Work out the finished part from the listing and answer in its coordinate system (mm). Face numbers are marked on the shaded views. A direction names the side the tool comes from. Coordinates: 2 decimals unless noted, no trailing zeros. Write each loop counter-clockwise with the first axis right and the second up, starting at its lowest first coordinate (ties: lowest second). Pieces come first, ordered by that corner, then holes. Notation, with made-up numbers: (24, 53) - (68, 53) arc R25 ccw to (68, 73) - close; hole circle Ø1 at (37.25, 29). An arc over 180 degrees is marked (long way). One line per item, written item: value.
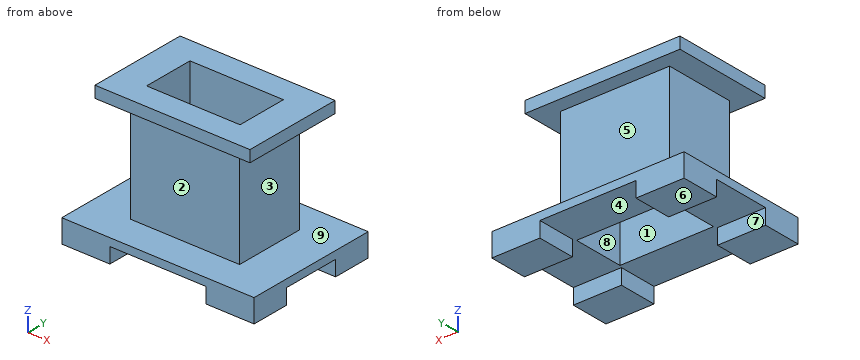
```python
from build123d import *

# Parameters (mm, degrees)
F0_W      = 127
F0_H      = 88.9
F1_DEPTH  = 15.24
F2_W      = 63.5
F2_H      = 10.16
F3_DEPTH  = 88.9
F4_W      = 38.1
F4_H      = 10.16
F5_DEPTH  = 127
F6_W      = 71.8820020556
F6_H      = 46.4872904122
F7_DEPTH  = 76.2
F8_W      = 61.7219954729
F8_H      = 33.7767079473
F9_DEPTH  = 101.6
F10_W     = 102.3619994521
F10_H     = 66.2887096405
F10_W_2   = 71.8820020556
F10_H_2   = 46.4872904122
F11_DEPTH = 7.62


with BuildPart() as f1:
    # F0 (on Top) → F1 (new body)
    with BuildSketch(Plane.XY):
        Rectangle(F0_W, F0_H)
    extrude(amount=-F1_DEPTH)

    # F2 (on face) → F3 (cut)
    with BuildSketch(Plane.XZ.offset(44.45)):
        with Locations((0, -10.16)):
            Rectangle(F2_W, F2_H)
    extrude(amount=-F3_DEPTH, mode=Mode.SUBTRACT)

    # F4 (on face) → F5 (cut)
    with BuildSketch(Plane(origin=(-63.5, 0, 0), x_dir=(0, -1, 0), z_dir=(-1, 0, 0))):
        with Locations((0, -10.16)):
            Rectangle(F4_W, F4_H)
    extrude(amount=-F5_DEPTH, mode=Mode.SUBTRACT)

    # F6 (on face) → F7 (join)
    with BuildSketch(Plane.XY):
        Rectangle(F6_W, F6_H)
    extrude(amount=F7_DEPTH)

    # F8 (on face) → F9 (cut)
    with BuildSketch(Plane.XY.offset(76.2)):
        Rectangle(F8_W, F8_H)
    extrude(amount=-F9_DEPTH, mode=Mode.SUBTRACT)

    # F10 (on face) → F11 (join)
    with BuildSketch(Plane.XY.offset(76.2)):
        Rectangle(F10_W, F10_H)
        Rectangle(F10_W_2, F10_H_2, mode=Mode.SUBTRACT)
    extrude(amount=-F11_DEPTH)


solid = f1.part
```
Item 1: Which of the six approach directions +Z, -Z, +X, -X, +Y, -Y give full straight-line access (tool end or side, diameter ignored) to the marked faces 5, 6, 7, 8 and 9?
Evaluation:
face 5: +X, -X, +Y
face 6: -Z, +X, -X, +Y, -Y
face 7: -Z, +X, -X
face 8: +Z, -Z
face 9: none
Item 2: Section C-C, the plane y = 12 is taken. Determine the outline of the cut face in (x, z).
Evaluation:
outline: (-63.5, -5.08) - (-30.86, -5.08) - (-30.86, 76.2) - (-51.18, 76.2) - (-51.18, 68.58) - (-35.94, 68.58) - (-35.94, 0) - (-63.5, 0) - close; (30.86, -5.08) - (63.5, -5.08) - (63.5, 0) - (35.94, 0) - (35.94, 68.58) - (51.18, 68.58) - (51.18, 76.2) - (30.86, 76.2) - close
Item 3: Given pin 1 (2.5 mm diameter, centred on x = -5.5, z = 72.5, fed in from -Y); pin 2 (3 mm diameter, centred on x = -22.5, y = -15, fed in from +Z); pin 3 (12 mm diameter, centred on x = 37.5, z = 40, fed in from -Y); pin 4 (20 mm diameter, centred on x = -10.5, y = 14.5, fed in from -Z), each flat-ended and moving along its own axis, determine where each tip first touches the part or whether it passes through.
Evaluation:
pin 1: stops at y = -33.14
pin 2: passes through
pin 3: stops at y = -23.24
pin 4: stops at z = -5.08
Item 4: Section A-A, the plane z = -8 is taken. Determine the outline of the cut face in (x, y).
Evaluation:
outline: (-63.5, -44.45) - (-31.75, -44.45) - (-31.75, -19.05) - (-63.5, -19.05) - close; (-63.5, 19.05) - (-31.75, 19.05) - (-31.75, 44.45) - (-63.5, 44.45) - close; (31.75, -44.45) - (63.5, -44.45) - (63.5, -19.05) - (31.75, -19.05) - close; (31.75, 19.05) - (63.5, 19.05) - (63.5, 44.45) - (31.75, 44.45) - close
Item 5: Consider probe 1 along Z at (x, y) = (-47.5, -26); probe 2 along Y at (x, z) = (12.5, 30.5); probe 3 along X at (y, z) = (-11, 16.5). Determine where each line is inside the solid, lowest interval first.
Evaluation:
probe 1: z = -15.24 to 0, 68.58 to 76.2
probe 2: y = -23.24 to -16.89, 16.89 to 23.24
probe 3: x = -35.94 to -30.86, 30.86 to 35.94
Item 6: Determine the mould class of the marked faces 1, 2, 3 and 4 for opening direction Y: +Y half, -Y half, draft (parallel to the pull), parting line (faces both ways), or undercut.
Evaluation:
face 1: undercut
face 2: -Y half
face 3: draft
face 4: undercut
Item 7: Section D-D, the plane z = 32.5 is taken. Determine the outline of the cut face in (x, y).
Evaluation:
outline: (-35.94, -23.24) - (35.94, -23.24) - (35.94, 23.24) - (-35.94, 23.24) - close; hole (-30.86, -16.89) - (30.86, -16.89) - (30.86, 16.89) - (-30.86, 16.89) - close
Item 8: Section B-B, the plane x = -43.5 is taken. Determine the outline of the cut face in (y, z).
Evaluation:
outline: (-44.45, -15.24) - (-19.05, -15.24) - (-19.05, -5.08) - (19.05, -5.08) - (19.05, -15.24) - (44.45, -15.24) - (44.45, 0) - (-44.45, 0) - close; (-33.14, 68.58) - (33.14, 68.58) - (33.14, 76.2) - (-33.14, 76.2) - close
